```python
from build123d import *

# Parameters (mm, degrees)
F0_R     = 3.175
F1_DEPTH = 16.51
F3_D     = 3.4544
F3_DEPTH = 5.08
F3_TIP   = 1.0378064612
F4_SIZE  = 0.254


with BuildPart() as f1:
    # F0 (on Front) → F1 (new body)
    with BuildSketch(Plane.XZ):
        Circle(F0_R)
    extrude(amount=F1_DEPTH)

    # F3
    with Locations(Plane.XZ.offset(16.51)):
        with Locations((0, 0)):
            Hole(F3_D / 2, depth=F3_DEPTH)
            with Locations((0, 0, -(F3_DEPTH + F3_TIP / 2))):  # 118° drill point
                Cone(0, F3_D / 2, F3_TIP, mode=Mode.SUBTRACT)

    # F4
    f4_edges = [f1.edges().sort_by_distance(p)[0] for p in [
        (-3.175, 0, 0),
    ]]
    chamfer(f4_edges, length=F4_SIZE)


solid = f1.part
```
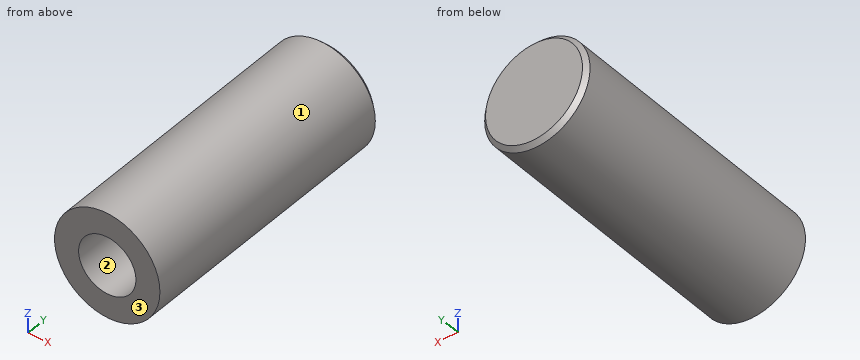
Work out the finished part from the listing and answer in its coordinate system (mm). Face numbers are marked on the shaded views. Give positions to 0.01 mm unless a question says otherwise; leave off trailing zeros. Loops run counter-clockwise (first coordinate to the right, second up) from the corner with the lowest first, then second, coordinate; pieces in that order, holes last. Notation, with made-up numbers: (15.5, 13.25) -> (71.5, 13.25) arc R21 cw to (71.5, 27.25) -> close; hole circle Ø3 at (38.25, -27.5). An arc over 180 degrees is marked (long way). Put each result on its own line as item: value. Start each with the question number.
Item 1: The mould has two halves that part along X. Classify the marked faces 1, 2 and 3: released by +X, released by -X, zero draft, split by the parting line, or undercut.
Item 2: The part is cut by section A-A (y = -13). Give the vertices of the cut face in (x, z) (3 decimals), then the cut area to 3 significant figures.
Item 3: The part is cut by section B-B (y = -3.25). Give the vertices of the cut face in (x, z) (3 decimals).
Item 4: Find the intervals of material crossed by L1, parallel to Z at x = 0, y = -13.5 (3 decimals); L2, parallel to X at y = -1.75, z = -1.25; L3, parallel to Z at x = -0.5, y = -15, in increasing order. Write a range as [from, to].
Answers below:
1. face 1: split by the parting line
1. face 2: undercut
1. face 3: zero draft
2. outline: circle Ø6.35 at (0, 0); hole circle Ø3.454 at (0, 0)
2. area: 22.3 mm2
3. outline: circle Ø6.35 at (0, 0)
4. L1: [-3.175, -1.727], [1.727, 3.175]
4. L2: [-2.92, 2.92]
4. L3: [-3.14, -1.65], [1.65, 3.14]
